Can you work these out from the model? Positions are in its coordinate system, mm. Give positions to 0.01 mm unless a question says otherwise; leave off trailing zeros. Loops run counter-clockwise (first coordinate to the right, second up) from the corner with the lowest first, then second, coordinate; pieces in that order, holes last. Notation, with made-up numbers: M 27,53.25 L 74,53.25 A15 ccw 74,71.25 Z; hole C -15.75,66.25 d1. An arc over 180 degrees is marked long. Put each result on its own line as item: value. Start each with the question number.
1) For P1, Ø3, axis at x = 65.5, z = 31.5, coming from the -Y side, with a flat end and sliding along its axis, tell me the tip position at first contact or that it passes through.
2) Imagine slicing it at B-B (y = 0.9). Write out the boundary of the cut face in (x, z), then the cut area to 3 significant figures.
3) Imagine slicing it at D-D (x = 90). Write out the boundary of the cut face in (y, z), then the cut area to 3 significant figures.
4) Imagine slicing it at A-A (x = 36.5). Write out the boundary of the cut face in (y, z), then the cut area to 3 significant figures.
5) Imagine slicing it at C-C (z = 25). Write out the boundary of the cut face in (x, y), then the cut area to 3 significant figures.
6) Please list where these lines run through material, in increasing order: line 1 along X through (y, z) = (2.35, 25); line 2 along Z through (x, y) = (31.5, 0.7); line 3 along Z through (x, y) = (90, 1.5). Write a range as from..to.
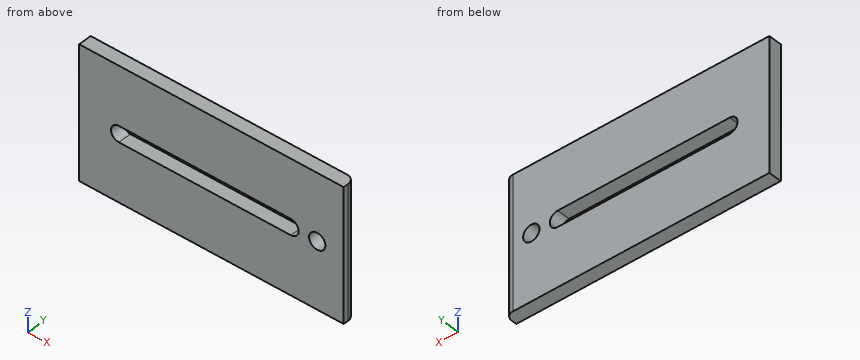
Autodesk Inventor part; units mm, degrees
ref_plane "Work Plane1" through (100, 5, 5) normal (0, 0, -1) x (-1, 0, 0)
ref_plane "Work Plane2" through (0, 5, 45) normal (0, 0, 1) x (1, 0, 0)
ref_plane "YZ Plane" through (0, 0, 0) normal (1, 0, 0) x (0, 1, 0)
sketch "Sketch1" plane through (0, 0, 0) normal (0, 1, 0) x (-1, 0, 0)
  line L0 (0, 0) -> (-100, 0)
  line L1 (-100, 0) -> (-100, 50)
  line L2 (-100, 50) -> (0, 50)
  line L3 (0, 50) -> (0, 0)
  point P0 (-50, 0)
  point P1 (-90, 25)
  dimension "d0" = 100
  dimension "d1" = 50
  dimension "d24" = 10
  dimension "d25" = 25
extrude "Extrusion1" add sketch "Sketch1" along normal blind 5
sketch "Sketch2" plane through (0, 5, 0) normal (0, 1, 0) x (1, 0, 0)
  line L0 (0, -50) -> (100, -50) construction
  line L1 (100, -50) -> (100, 0) construction
  line L2 (100, 0) -> (0, 0) construction
  line L3 (0, 0) -> (0, -50) construction
  line L4 (80, -25) -> (15, -25) construction
  arc A0 (80, -28) -> (80, -22) centre (80, -25) ccw
  arc A1 (15, -22) -> (15, -28) centre (15, -25) ccw
  line L5 (15, -22) -> (80, -22)
  line L6 (80, -28) -> (15, -28)
  point P0 (50, -50)
  dimension "d7" = 65
  dimension "d8" = 25
  dimension "d9" = 15
  dimension "d10" = 6
  dimension "dia" = 6
extrude "Extrusion2" cut sketch "Sketch2" against normal blind 5
sketch "Sketch5" plane through (0, 5, 0) normal (0, 1, 0) x (1, 0, 0)
  line L0 (0, -50) -> (100, -50)
  line L1 (100, -50) -> (100, 0)
  point P0 (0, 0)
  point P1 (90, -25)
  dimension "d33" = 25
  dimension "d34" = 10
hole "Hole1" at (90, 5, 25) direction (0, -1, 0) diameter 6.2 end through all
thread "Thread1"
ref_plane "Work Plane1" through (100, 5, 5) normal (0, 0, -1) x (-1, 0, 0)
ref_plane "Work Plane2" through (0, 5, 45) normal (0, 0, 1) x (1, 0, 0)
fillet "Fillet1" radius 3 1 edges at (100, 5, 25)
equation "\"d10\" = dia"
properties part number "Horonyrogzito"
Recorded:
1. P1: y = 0
2. outline: M 0,0 L 100,0 L 100,50 L 0,50 Z; hole M 15,22 L 80,22 A3 ccw 80,28 L 15,28 A3 ccw Z; hole C 90,25 d6.2
2. area: 4,550 mm²
3. outline: M 0,0 L 5,0 L 5,21.9 L 0,21.9 Z; M 0,28.1 L 5,28.1 L 5,50 L 0,50 Z
3. area: 219 mm²
4. outline: M 0,0 L 5,0 L 5,22 L 0,22 Z; M 0,28 L 5,28 L 5,50 L 0,50 Z
4. area: 220 mm²
5. outline: M 0,0 L 12,0 L 12,5 L 0,5 Z; M 83,0 L 86.9,0 L 86.9,5 L 83,5 Z; M 93.1,0 L 100,0 L 100,2 A3 ccw 97,5 L 93.1,5 Z
5. area: 112 mm²
6. line 1: 0..12, 83..86.9, 93.1..99.98
6. line 2: 0..22, 28..50
6. line 3: 0..21.9, 28.1..50
